Could you check a few things on this model? Use its own coordinates, in mm. Face numbers are marked on the shaded views. A direction names the side the tool comes from. Coordinates: 2 decimals unless noted, no trailing zeros. Loops run counter-clockwise (first coordinate to the right, second up) from the corner with the lowest first, then second, coordinate; pieces in that order, holes last.
from build123d import *

# Parameters (mm, degrees)
F1_DEPTH      = 8
F3_DEPTH      = 25
F3_DEPTH_BACK = 25
F4_W          = 16
F4_H          = 8
F5_DEPTH      = 10
F6_R          = 5
F7_R          = 5
F8_DEPTH      = 0.4


with BuildPart() as f1:
    # F0 (on Top) → F1 (new body)
    with BuildSketch(Plane.XY):
        with BuildLine():
            Line((-1, 0), (0, 0))
            Line((0, 0), (5, 0))
            Line((5, 0), (5, 14))
            Line((5, 14), (-18, 14))
            Line((-18, 14), (-18, 9))
            Line((-18, 9), (0, 9))
            Line((0, 9), (0, 3))
            Line((0, 3), (-1, 3))
            ThreePointArc((-1, 3), (-2.5, 1.5), (-1, 0))
        make_face()
    extrude(amount=F1_DEPTH)

    # F2 (on face) → F3 (cut, two sides)
    with BuildSketch(Plane(origin=(0, 14, 0), x_dir=(-1, 0, 0), z_dir=(0, 1, 0))) as f3_sk:
        Polygon((15.3, 2.2838863602), (15.3, 5.7318202537), (14.9282596673, 5.7318202537), (13.4143294991, 4.8903837167), (13.3860698318, 3.1585634629), (14.8717403327, 2.2681797463), (15.2717403327, 2.2681797463), align=None)
        Polygon((15.3282596673, 5.7318202537), (15.3, 5.7318202537), (15.3, 2.2838863602), (16.7856705009, 3.1096162833), (16.8139301682, 4.8414365371), align=None)
    extrude(amount=-F3_DEPTH, mode=Mode.SUBTRACT)
    extrude(f3_sk.sketch, amount=F3_DEPTH_BACK, mode=Mode.SUBTRACT)

    # F4 (on face) → F5 (join)
    with BuildSketch(Plane(origin=(0, 14, 0), x_dir=(-1, 0, 0), z_dir=(0, 1, 0))):
        with Locations((3, 4)):
            Rectangle(F4_W, F4_H)
    extrude(amount=F5_DEPTH)

    # F6
    f6_edges = [f1.edges().sort_by_distance(p)[0] for p in [
        (5, 24, 4),
        (-11, 24, 4),
    ]]
    fillet(f6_edges, radius=F6_R)

    # F7
    f7_edges = [f1.edges().sort_by_distance(p)[0] for p in [
        (5, 0, 4),
    ]]
    fillet(f7_edges, radius=F7_R)

    # F8 (add): a face of the model
    f8_faces = [f1.faces().sort_by_distance(p)[0] for p in [
        (-18, 11.5, 4),
    ]]
    extrude(f8_faces, amount=F8_DEPTH)


solid = f1.part
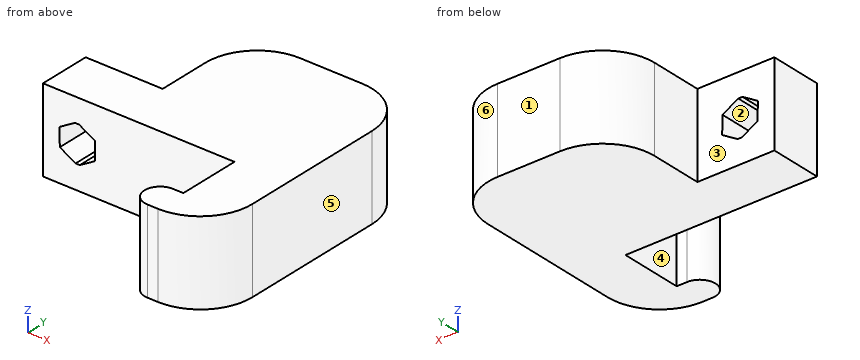
(1) Imagine slicing it at B-B, the plane z = 3.5. Write out the boundary of the cut face in (x, y), and give its area (3 significant figures).
Answers:
outline: (-18.4, 9) - (-16.79, 9) - (-16.79, 14) - (-18.4, 14) - close; (-13.39, 9) - (0, 9) - (0, 3) - (-1, 3) arc R1.5 ccw to (-1, 0) - (0, 0) arc R5 ccw to (5, 5) - (5, 19) arc R5 ccw to (0, 24) - (-6, 24) arc R5 ccw to (-11, 19) - (-11, 14) - (-13.39, 14) - close
area: 295 mm2
(2) For pin 1 (2.5 mm diameter, centred on y = 16, z = 6, fed in from -X), with a flat end and sliding along its axis, tell me the tip position at first contact or that it passes through.
Answers:
pin 1: stops at x = -11
(3) We'd pull the mould along Y, two halves only. Please class the marked faces 4, 5 and 6: +Y half, -Y half, draft (parallel to the pull), parting line (faces both ways), or undercut.
Answers:
face 4: undercut
face 5: draft
face 6: +Y half
(4) Which directions (+Z, -Z, +X, -X, +Y, -Y) give clear straight access to the entire face, cutting with the end or side of a thin tool? Please do the marked faces 1, 2 and 3.
Answers:
face 1: +Z, -Z, +X, -X, +Y
face 2: +Y, -Y
face 3: +Z, -Z, -X, +Y
(5) Imagine slicing it at D-D, the plane y = 18. Write out the boundary of the cut face in (x, z), and give its area (3 significant figures).
Answers:
outline: (-11, 0) - (5, 0) - (5, 8) - (-11, 8) - close
area: 128 mm2
(6) I need wall thicknesses on probe 1 along X at (y, z) = (11.5, 3.25); probe 2 along Y at (x, z) = (-1, 0.5); probe 3 along X at (y, z) = (8, 6). Which ranges of each line are inside material? Lowest first, please.
Answers:
probe 1: x = -18.4 to -16.79, -13.39 to 5
probe 2: y = 0 to 3, 9 to 24
probe 3: x = 0 to 5
(7) Imagine slicing it at A-A, the plane y = 10. Write out the boundary of the cut face in (x, z).
Answers:
outline: (-18.4, 0) - (5, 0) - (5, 8) - (-18.4, 8) - close; hole (-16.81, 4.84) - (-16.79, 3.11) - (-15.27, 2.27) - (-14.87, 2.27) - (-13.39, 3.16) - (-13.41, 4.89) - (-14.93, 5.73) - (-15.33, 5.73) - close
(8) Imagine slicing it at C-C, the plane x = 3. Write out the boundary of the cut face in (y, z), and give its area (3 significant figures).
Answers:
outline: (1, 0) - (23, 0) - (23, 8) - (1, 8) - close
area: 176 mm2
